from build123d import *

# Parameters (mm, degrees)
SKETCH1_R           = 30
BOSS_EXTRUDE1_DEPTH = 75
SKETCH2_R           = 3.5
SKETCH2_R_2         = 2.5
CUT_EXTRUDE1_DEPTH  = 10
SKETCH3_R           = 16
BOSS_EXTRUDE2_DEPTH = 2


with BuildPart() as part:
    # Sketch1 → Boss-Extrude1 (new body)
    with BuildSketch(Plane.XY):
        Circle(SKETCH1_R)
    extrude(amount=BOSS_EXTRUDE1_DEPTH)

    # Sketch2 → Cut-Extrude1 (cut)
    with BuildSketch(Plane.XY.offset(75)):
        with Locations((0, 25)):
            Circle(SKETCH2_R)
        with Locations((17.67766953, 17.67766953)):
            Circle(SKETCH2_R_2)
        with Locations(Location((-17.67766953, 17.67766953, 0), (0, 0, 180))):
            Circle(SKETCH2_R_2)
        with Locations(Location((17.67766953, -17.67766953, 0), (0, 0, 180))):
            Circle(SKETCH2_R_2)
        with Locations((-17.67766953, -17.67766953)):
            Circle(SKETCH2_R_2)
        with Locations(Location((25, 0, 0), (0, 0, 180))):
            Circle(SKETCH2_R)
        with Locations(Location((-25, 0, 0), (0, 0, 180))):
            Circle(SKETCH2_R)
        with Locations((0, -25)):
            Circle(SKETCH2_R)
    extrude(amount=-CUT_EXTRUDE1_DEPTH, mode=Mode.SUBTRACT)

    # Sketch3 → Boss-Extrude2 (add)
    with BuildSketch(Plane.XY.offset(75)):
        Circle(SKETCH3_R)
    extrude(amount=BOSS_EXTRUDE2_DEPTH)


solid = part.part
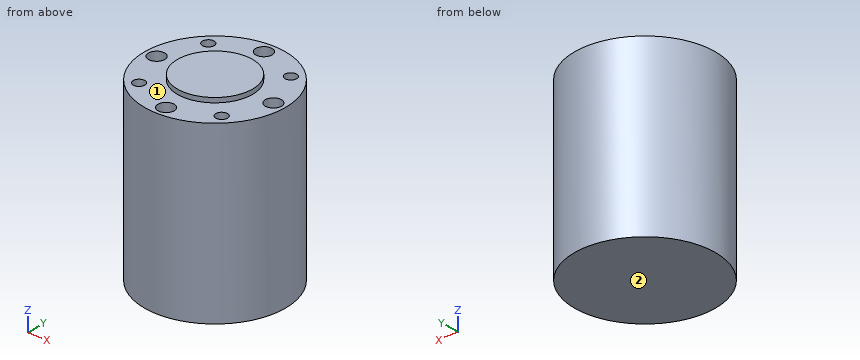
Design review of the part built by this model. Coordinates are the model's own, in mm. Face numbers are marked on the shaded views. A direction names the side the tool comes from. Give positions to 0.01 mm unless a question says otherwise; leave off trailing zeros. Loops run counter-clockwise (first coordinate to the right, second up) from the corner with the lowest first, then second, coordinate; pieces in that order, holes last. Notation, with made-up numbers: (10.25, 70.25) - (24.25, 70.25) arc R24 cw to (24.25, 87.25) - close; hole circle Ø3 at (-17.5, 89.5). An arc over 180 degrees is marked (long way). Use CSV: the item, a comma, the result in double quotes. Start each with the question number.
1. Add section D-D (y = 9.5). State the section outline as (x, z) points.
2. Machinability: for the marked faces 1 and 2, which of the approach directions +Z, -Z, +X, -X, +Y, -Y give a long, thin tool a straight path to every point of the face, cutting with its end or side? Answer none if there is none.
3. Add section C-C (z = 31). State the section outline as (x, y) points.
4. Insertion check: P1, Ø12, axis at x = -17.5, z = 17, coming from the -Y side; P2, Ø2, axis at x = 1.5, y = 26, coming from the +Z side; P3, Ø2, axis at x = 2, z = 68.5, coming from the -Y side. Each pin has a flat end and moves straight along its axis. Give the tip position at first contact, or say it passes through.
5. Add section A-A (x = 0). State the section outline as (y, z) points.
6. Wall thickness on L1, parallel to Y at x = 16.5, z = 70.5; L2, parallel to Z at x = -6.5, y = 26.5; L3, parallel to Y at x = -1, z = 68: over which ranges is each line inside the solid? List them lowest first.
Results found:
1,outline,"(-28.46, 0) - (28.46, 0) - (28.46, 75) - (12.87, 75) - (12.87, 77) - (-12.87, 77) - (-12.87, 75) - (-28.46, 75) - close"
2,face 1,"+Z"
2,face 2,"-Z, +X, -X, +Y, -Y"
3,outline,"circle Ø60 at (0, 0)"
4,P1,"stops at y = -27.71"
4,P2,"stops at z = 65"
4,P3,"stops at y = -29.98"
5,outline,"(-30, 0) - (30, 0) - (30, 75) - (28.5, 75) - (28.5, 65) - (21.5, 65) - (21.5, 75) - (16, 75) - (16, 77) - (-16, 77) - (-16, 75) - (-21.5, 75) - (-21.5, 65) - (-28.5, 65) - (-28.5, 75) - (-30, 75) - close"
6,L1,"y = -25.05 to -19.88, -15.47 to 15.47, 19.88 to 25.05"
6,L2,"z = 0 to 75"
6,L3,"y = -29.98 to -28.35, -21.65 to 21.65, 28.35 to 29.98"
